Autodesk Inventor part; units mm, degrees
sketch "Sketch1" plane through (0, 0, 0) normal (0, 0, 1) x (1, 0, 0)
  line L0 (-4.55, 7.5) -> (4.55, 7.5)
  line L1 (4.55, 7.5) -> (4.55, -7.5)
  line L2 (4.55, -7.5) -> (-4.55, -7.5)
  line L3 (-4.55, -7.5) -> (-4.55, 7.5)
  line L4 (-4.55, 7.5) -> (4.55, -7.5) construction
  line L5 (4.55, 7.5) -> (-4.55, -7.5) construction
  line L6 (-2.05, -2.05) -> (2.05, -2.05)
  line L7 (2.05, -2.05) -> (2.05, 2.05)
  line L8 (2.05, 2.05) -> (-2.05, 2.05)
  line L9 (-2.05, 2.05) -> (-2.05, -2.05)
  line L10 (-2.05, -2.05) -> (2.05, 2.05) construction
  line L11 (2.05, -2.05) -> (-2.05, 2.05) construction
  line L12 (-4.55, 6) -> (-4.55, 7.5)
  line L13 (-4.55, -6) -> (-4.55, -7.5)
  line L14 (4.55, 6) -> (4.55, 7.5)
  line L15 (4.55, -6) -> (4.55, -7.5)
  point P0 (0, 0)
  point P1 (16.55, 6)
  dimension "d1" = 9.1
  dimension "d2" = 4.1
  dimension "d3" = 4.1
extrude "Extrusion1" add sketch "Sketch1" along normal blind 12
sketch "Sketch2" plane through (0, 0, 12) normal (0, 0, 1) x (1, 0, 0)
  line L0 (4.55, 7.5) -> (-4.55, 7.5)
  line L1 (-4.55, 7.5) -> (-1.7, 7.5)
  line L2 (-1.7, 7.5) -> (-1.7, 14.5)
  line L3 (-1.7, 14.5) -> (-4.55, 14.5)
  line L4 (-4.55, 14.5) -> (-4.55, 7.5)
  line L5 (1.7, 7.5) -> (4.55, 7.5)
  line L6 (4.55, 7.5) -> (4.55, 14.5)
  line L7 (4.55, 14.5) -> (1.7, 14.5)
  line L8 (1.7, 14.5) -> (1.7, 7.5)
  point P0 (0, 0)
  point P1 (16.55, 7.5)
  point P2 (-16.55, 7.5)
  dimension "d15" = 2.85
  dimension "d16" = 2.85
  dimension "d17" = 7
  dimension "d18" = 7
  dimension "d19" = 1.7
  dimension "d20" = 1.7
extrude "Extrusion2" add sketch "Sketch2" against normal up to surface (12 mm away)
sketch "Sketch5" plane through (0, 0, 0) normal (0, 0, -1) x (-1, 0, 0)
  line L0 (-2.05, 5.05) -> (2.05, 5.05)
  line L1 (2.05, 5.05) -> (2.05, 3.55)
  line L2 (2.05, 3.55) -> (-2.05, 3.55)
  line L3 (-2.05, 3.55) -> (-2.05, 5.05)
  line L4 (-2.05, -3.55) -> (2.05, -3.55)
  line L5 (2.05, -3.55) -> (2.05, -5.05)
  line L6 (2.05, -5.05) -> (-2.05, -5.05)
  line L7 (-2.05, -5.05) -> (-2.05, -3.55)
  line L8 (2.05, 2.05) -> (-2.05, 2.05)
  line L9 (2.05, -2.05) -> (2.05, 2.05)
  line L10 (-2.05, -2.05) -> (2.05, -2.05)
  point P0 (0, 0)
  dimension "d31" = 4.1
  dimension "d32" = 4.1
  dimension "d33" = 1.5
  dimension "d34" = 1.5
  dimension "d35" = 1.5
  dimension "d36" = 1.5
extrude "Extrusion4" cut sketch "Sketch5" against normal through all
sketch "Sketch6" plane through (0, 0, 12) normal (0, 0, 1) x (1, 0, 0)
  line L0 (-4.55, 14.5) -> (-4.55, -7.5)
  line L1 (-4.55, -7.5) -> (4.55, -7.5)
  line L2 (-4.55, -3.55) -> (4.55, -3.55)
  line L3 (4.55, -3.55) -> (4.55, -7.5)
  line L4 (4.55, -7.5) -> (-4.55, -7.5)
  line L5 (-4.55, -7.5) -> (-4.55, -3.55)
  line L6 (-2.05, -3.55) -> (2.05, -3.55)
  point P0 (0, 0)
  dimension "d42" = 0
extrude "Extrusion5" cut sketch "Sketch6" against normal through all
fillet "Fillet3" radius 2 6 edges at (4.55, -3.55, 6) (-4.55, -3.55, 6) (3.125, 14.5, 12) (-3.125, 14.5, 12) (-3.125, 14.5, 0) (3.125, 14.5, 0)
equation "\"d31\" = d32"
properties part number "fuselage_honeycomb_interface_v2"
Source: CAD feature listing. Evaluate the final solid. Frame: model axes, mm. A direction names the side the tool comes from. Give positions to 0.01 mm unless a question says otherwise; leave off trailing zeros. Loops run counter-clockwise (first coordinate to the right, second up) from the corner with the lowest first, then second, coordinate; pieces in that order, holes last. Notation, with made-up numbers: (32, 13) - (36, 13) arc R24 cw to (36, 34) - close; hole circle Ø3 at (-24, -25.75). An arc over 180 degrees is marked (long way). Use CSV: the item, a comma, the result in double quotes.
1) Line query: line 1 (Y direction, x = -0.25, z = 7.75); line 2 (Y direction, x = -2, z = 10); line 3 (X direction, y = 12, z = 9.5). Output: solid intervals per line, ascending.
Worked out:
line 1,"y = -3.55 to -2.05, 2.05 to 3.55, 5.05 to 7.5"
line 2,"y = -3.55 to -2.05, 2.05 to 3.55, 5.05 to 14.5"
line 3,"x = -4.55 to -1.7, 1.7 to 4.55"
2) Cut plane D-D (y = 13). Output: boundary loops of the cut face in (x, z), and give its area (3 significant figures).
Worked out:
outline,"(-4.55, 0.06) - (-1.7, 0.06) - (-1.7, 11.94) - (-4.55, 11.94) - close; (1.7, 0.06) - (4.55, 0.06) - (4.55, 11.94) - (1.7, 11.94) - close"
area,"67.7 mm^2"
3) Cut plane A-A (y = -0.75). Output: boundary loops of the cut face in (x, z), and give its area (3 significant figures).
Worked out:
outline,"(-4.55, 0) - (-2.05, 0) - (-2.05, 12) - (-4.55, 12) - close; (2.05, 0) - (4.55, 0) - (4.55, 12) - (2.05, 12) - close"
area,"60.0 mm^2"
4) Mould query, pull axis Y, two halves, no side actions, for faces 4 (the cylindrical face through (3.11, 13.9, 11.43)), 5 (the flat face through (1.7, 11, 6)), 6 (the flat face through (0, -2.05, 6)). Classes: +Y half, -Y half, draft (parallel to the pull), parting line (faces both ways), or undercut.
Worked out:
face 4,"+Y half"
face 5,"draft"
face 6,"undercut"
5) Cut plane B-B (z = 5.25). Output: boundary loops of the cut face in (x, y).
Worked out:
outline,"(-4.55, -1.55) arc R2 ccw to (-2.55, -3.55) - (2.55, -3.55) arc R2 ccw to (4.55, -1.55) - (4.55, 14.5) - (1.7, 14.5) - (1.7, 7.5) - (-1.7, 7.5) - (-1.7, 14.5) - (-4.55, 14.5) - close; hole (-2.05, -2.05) - (2.05, -2.05) - (2.05, 2.05) - (-2.05, 2.05) - close; hole (-2.05, 3.55) - (2.05, 3.55) - (2.05, 5.05) - (-2.05, 5.05) - close"
6) Cut plane C-C (x = -0.5). Output: boundary loops of the cut face in (y, z), and give its area (3 significant figures).
Worked out:
outline,"(-3.55, 0) - (-2.05, 0) - (-2.05, 12) - (-3.55, 12) - close; (2.05, 0) - (3.55, 0) - (3.55, 12) - (2.05, 12) - close; (5.05, 0) - (7.5, 0) - (7.5, 12) - (5.05, 12) - close"
area,"65.4 mm^2"
7) Pin query (flat end, axial travel): P1, Ø2, axis at x = -0.5, z = 6.5, coming from the +Y side. Return the tip coordinate at first contact, or that it passes through.
Worked out:
P1,"stops at y = 7.5"
8) Set-up query: faces 1 (the flat face through (2.05, 4, 6)), 2 (the flat face through (-1.7, 11, 6)), 3 (the cylindrical face through (-3.95, -2.98, 5.92)). Return all of +Z, -Z, +X, -X, +Y, -Y with unobstructed straight access to the full face (end or side cutting, diameter ignored); none if empty.
Worked out:
face 1,"+Z, -Z"
face 2,"+Z, -Z, +Y"
face 3,"+Z, -Z, -X, -Y"
